Here's how the part is built. I have some questions about the finished solid (model axes, mm). A direction names the side the tool comes from. Coordinates: 2 decimals unless noted, no trailing zeros. Loops run counter-clockwise (first coordinate to the right, second up) from the corner with the lowest first, then second, coordinate; pieces in that order, holes last. Notation, with made-up numbers: (-25, 27) -> (3, 27) arc R31 ccw to (3, 53) -> close; hole circle Ø6 at (76.5, 49.25). An arc over 180 degrees is marked (long way). Answer as a JSON object with one key per item and string values. Group by question number.
1) I'm going to push flat-ended pins straight in: pin 1 (4 mm diameter, centred on y = 10.5, z = -0.5, fed in from +X); pin 2 (2.5 mm diameter, centred on x = 9.5, z = 0, fed in from +Y). Where does each tip first touch, or does it pass through?
2) I want a section at D-D (y = -2.25). Write out the boundary of the cut face in (x, z), then the cut area to 3 significant figures.
3) I want a section at A-A (x = 0). Write out the boundary of the cut face in (y, z), then the cut area to 3 significant figures.
4) If we mould it in two halves opening along Y, with no side actions, what happens to faces 1 (the cylindrical face through (11, 10, 0)), 2 (the flat face through (0, 1.75, 0))? For each: +Y half, -Y half, draft (parallel to the pull), parting line (faces both ways), or undercut.
5) I need wall thicknesses on probe 1 along X at (y, z) = (-10.45, 0); probe 2 along X at (y, z) = (9.3, 0); probe 3 along Y at (x, z) = (-4.9, -3). Which ranges of each line are inside material? Lowest first, please. Write a range as [from, to].
6) Which directions (+Z, -Z, +X, -X, +Y, -Y) give clear straight access to the entire face, cutting with the end or side of a thin tool? Please do faces 3 (the cylindrical face through (-11, -10, 0)), 4 (the flat face through (-2, -8, -2)), 5 (the flat face through (2, 8, -2)), 6 (the flat face through (12, 10, 0)).
7) I want a section at C-C (y = -10.5). Write out the boundary of the cut face in (x, z), then the cut area to 3 significant figures.
8) I want a section at B-B (z = -3.5). Write out the boundary of the cut face in (x, y), then the cut area to 3 significant figures.
```python
from build123d import *

# Parameters (mm, degrees)
SKIZZE1_W                            = 24
SKIZZE1_H                            = 26
AUFSATZ_LINEAR_AUSTRAGEN1_DEPTH      = 10
SCHNITT_LINEAR_AUSTRAGEN1_DEPTH      = 21.322401433
SCHNITT_LINEAR_AUSTRAGEN2_DEPTH      = 21.322401433
SCHNITT_LINEAR_AUSTRAGEN3_DEPTH      = 21.322401433
SKIZZE5_W                            = 4
SKIZZE5_H                            = 10
SKIZZE6_W                            = 4
SKIZZE6_H                            = 10
F_2_3_2_3_DURCHMESSER_BOHRUNG1_D     = 2.3
F_2_3_2_3_DURCHMESSER_BOHRUNG1_DEPTH = 24
SKIZZE9_W                            = 2.1
SKIZZE9_H                            = 5
F_3_0_3_DURCHMESSER_BOHRUNG1_D       = 3
F_3_0_3_DURCHMESSER_BOHRUNG1_DEPTH   = 5
SKIZZE13_W                           = 2.1
SKIZZE13_H                           = 5
F_3_0_3_DURCHMESSER_BOHRUNG2_D       = 3
F_3_0_3_DURCHMESSER_BOHRUNG2_DEPTH   = 5
FASE1_SIZE                           = 0.25
SENSORKABEL_START                    = -35
SKIZZE24_R                           = 1.15
SENSORKABEL_DEPTH                    = 35


with BuildPart() as part:
    # Skizze1 → Aufsatz-Linear austragen1 (new body)
    with BuildSketch(Plane.XY.offset(5)):
        Rectangle(SKIZZE1_W, SKIZZE1_H)
    extrude(amount=-AUFSATZ_LINEAR_AUSTRAGEN1_DEPTH)

    # Skizze2 → Schnitt-Linear austragen1 (cut, through all)
    with BuildSketch(Plane(origin=(0, 0, -5), x_dir=(-1, 0, 0), z_dir=(0, 0, -1))):
        with BuildLine():
            Line((12, -8), (12, -5))
            Line((12, -5), (-8, -5))
            ThreePointArc((-8, -5), (-9.5, -6.5), (-8, -8))
            Line((-8, -8), (12, -8))
        make_face()
    extrude(amount=-SCHNITT_LINEAR_AUSTRAGEN1_DEPTH, mode=Mode.SUBTRACT)

    # Skizze3 → Schnitt-Linear austragen2 (cut, through all)
    with BuildSketch(Plane(origin=(0, 0, -5), x_dir=(-1, 0, 0), z_dir=(0, 0, -1))):
        with BuildLine():
            Line((-12, 8), (-12, 5))
            Line((-12, 5), (8, 5))
            ThreePointArc((8, 5), (9.5, 6.5), (8, 8))
            Line((8, 8), (-12, 8))
        make_face()
    extrude(amount=-SCHNITT_LINEAR_AUSTRAGEN2_DEPTH, mode=Mode.SUBTRACT)

    # Skizze4 → Schnitt-Linear austragen3 (cut, through all)
    with BuildSketch(Plane(origin=(0, 0, -5), x_dir=(-1, 0, 0), z_dir=(0, 0, -1))):
        with BuildLine():
            Line((-1.703126358, -1.75), (1.303126358, -1.75))
            ThreePointArc((1.303126358, -1.75), (0.9, 0), (1.303126358, 1.75))
            Line((1.303126358, 1.75), (-1.703126358, 1.75))
            ThreePointArc((-1.703126358, 1.75), (-1.3, 0), (-1.703126358, -1.75))
        make_face()
    extrude(amount=-SCHNITT_LINEAR_AUSTRAGEN3_DEPTH, mode=Mode.SUBTRACT)

    # Skizze5 → Schnitt-Rotation1 (revolve, cut)
    with BuildSketch(Plane(origin=(0, 0, 0), x_dir=(1, 0, 0), z_dir=(0, 1, 0))):
        with Locations((7.3, 0)):
            Rectangle(SKIZZE5_W, SKIZZE5_H)
    revolve(axis=Axis((5.3, 0, -5), (0, 0, 1)), mode=Mode.SUBTRACT)

    # Skizze6 → Schnitt-Rotation2 (revolve, cut)
    with BuildSketch(Plane(origin=(0, 0, 0), x_dir=(1, 0, 0), z_dir=(0, 1, 0))):
        with Locations((-2.9, 0)):
            Rectangle(SKIZZE6_W, SKIZZE6_H)
    revolve(axis=Axis((-4.9, 0, -5), (0, 0, 1)), mode=Mode.SUBTRACT)

    # Ø2.3 (2.3) Durchmesser Bohrung1
    with Locations(Plane.ZY.offset(12)):
        with Locations((0, 6.5)):
            Hole(F_2_3_2_3_DURCHMESSER_BOHRUNG1_D / 2, depth=F_2_3_2_3_DURCHMESSER_BOHRUNG1_DEPTH)

    # Skizze9 → M5 Gewindebohrung1 (revolve, cut)
    with BuildSketch(Plane(origin=(0, 8, 0), x_dir=(0, 0, -1), z_dir=(1, 0, 0))):
        with Locations((1.05, 2.5)):
            Rectangle(SKIZZE9_W, SKIZZE9_H)
    revolve(axis=Axis((0, 1.65, 0), (0, 1, 0)), mode=Mode.SUBTRACT)

    # Ø3.0 (3) Durchmesser Bohrung1
    with Locations(Plane(origin=(0, 13, 0), x_dir=(1, 0, 0), z_dir=(0, 1, 0))):
        with Locations((9.5, 0)):
            Hole(F_3_0_3_DURCHMESSER_BOHRUNG1_D / 2, depth=F_3_0_3_DURCHMESSER_BOHRUNG1_DEPTH)

    # Skizze13 → M5 Gewindebohrung2 (revolve, cut)
    with BuildSketch(Plane(origin=(0, -8, 0), x_dir=(0, 0, 1), z_dir=(1, 0, 0))):
        with Locations((1.05, 2.5)):
            Rectangle(SKIZZE13_W, SKIZZE13_H)
    revolve(axis=Axis((0, -1.65, 0), (0, -1, 0)), mode=Mode.SUBTRACT)

    # Ø3.0 (3) Durchmesser Bohrung2
    with Locations(Plane(origin=(0, -13, 0), x_dir=(-1, 0, 0), z_dir=(0, -1, 0))):
        with Locations((9.5, 0)):
            Hole(F_3_0_3_DURCHMESSER_BOHRUNG2_D / 2, depth=F_3_0_3_DURCHMESSER_BOHRUNG2_DEPTH)

    # Fase1
    fase1_edges = [part.edges().sort_by_distance(p)[0] for p in [
        (11, 13, 0),
        (-11, -13, 0),
    ]]
    chamfer(fase1_edges, length=FASE1_SIZE)

    # Skizze24 → Sensorkabel (add)
    with BuildSketch(Plane.ZY.offset(12).offset(SENSORKABEL_START)):
        with Locations((0, 6.5)):
            Circle(SKIZZE24_R)
    extrude(amount=SENSORKABEL_DEPTH)


solid = part.part
```
Determined:
{
 "1": {"pin 1": "x = 12", "pin 2": "y = 7.65"},
 "2": {"outline": "(-12, -5) -> (-8.21, -5) -> (-8.21, 5) -> (-12, 5) -> close; (-1.59, -5) -> (1.99, -5) -> (1.99, 5) -> (-1.59, 5) -> close; (8.61, -5) -> (12, -5) -> (12, 5) -> (8.61, 5) -> close", "area": "108 mm^2"},
 "3": {"outline": "(-13, -5) -> (-8, -5) -> (-8, -2.1) -> (-13, -2.1) -> close; (-13, 2.1) -> (-8, 2.1) -> (-8, 5) -> (-13, 5) -> close; (-5, -5) -> (-1.75, -5) -> (-1.75, 5) -> (-5, 5) -> close; (1.75, -5) -> (5, -5) -> (5, 5) -> (1.75, 5) -> close; circle Ø2.3 at (6.5, 0); (8, -5) -> (13, -5) -> (13, -2.1) -> (8, -2.1) -> close; (8, 2.1) -> (13, 2.1) -> (13, 5) -> (8, 5) -> close", "area": "127 mm^2"},
 "4": {"face 1": "draft", "face 2": "undercut"},
 "5": {"probe 1": "[-12, -11], [-8, -2.1], [2.1, 12]", "probe 2": "[-12, -2.1], [2.1, 8], [11, 12]", "probe 3": "[-13, -8], [-5, -4], [4, 5], [8, 13]"},
 "6": {"face 3": "-Y", "face 4": "+Z, -Z, -X", "face 5": "+Z, -Z, +X", "face 6": "+Z, -Z, +X, +Y"},
 "7": {"outline": "(-12, -5) -> (12, -5) -> (12, 5) -> (-12, 5) -> close; hole circle Ø3 at (-9.5, 0); hole circle Ø4.2 at (0, 0)", "area": "219 mm^2"},
 "8": {"outline": "(-12, -13) -> (12, -13) -> (12, 5) -> (-8, 5) arc R1.5 cw to (-8, 8) -> (12, 8) -> (12, 13) -> (-12, 13) -> (-12, -5) -> (8, -5) arc R1.5 cw to (8, -8) -> (-12, -8) -> close; hole (-1.3, -1.75) -> (1.7, -1.75) arc R4 ccw (long way) to (1.7, 1.75) -> (-1.3, 1.75) arc R4 ccw (long way) to start", "area": "388 mm^2"}
}
